Model file for the job. Use its own axes, mm. Round coordinates to 2 decimals unless told otherwise and drop trailing zeros. Order: outer loops, then holes, each group sorted by start corner. A loop starts at its lowest first (then second) coordinate and runs counter-clockwise, first axis right, second up. Notation, with made-up numbers: (62, 52.25) -> (84, 52.25) arc R19 cw to (84, 76.25) -> close; hole circle Ø5 at (-6.75, 43). An arc over 180 degrees is marked (long way). Answer as CSV lines item,"result".
Autodesk Inventor part; units mm, degrees
ref_plane "YZ Plane" through (0, 0, 0) normal (1, 0, 0) x (0, 1, 0)
ref_plane "XZ Plane" through (0, 0, 0) normal (0, 1, 0) x (-1, 0, 0)
ref_plane "XY Plane" through (0, 0, 0) normal (0, 0, 1) x (1, 0, 0)
sketch "Sketch1" plane through (0, 0, 0) normal (0, 0, 1) x (1, 0, 0)
  line L0 (-6.35, -3.6662) -> (-6.35, 3.6662)
  line L1 (-6.35, 3.6662) -> (0, 7.3323)
  line L2 (0, 7.3323) -> (6.35, 3.6662)
  line L3 (6.35, 3.6662) -> (6.35, -3.6662)
  line L4 (6.35, -3.6662) -> (0, -7.3323)
  line L5 (0, -7.3323) -> (-6.35, -3.6662)
  point P0 (0, 0)
  point P1 (0, 0)
  dimension "d0" = 12.7
extrude "Extrusion1" add sketch "Sketch1" along normal blind 73.0377
sketch "Sketch2" plane through (0, 0, 73.0377) normal (0, 0, 1) x (1, 0, 0)
  point P0 (0, 0)
  point P1 (0, 0)
hole "Hole1" at (0, 0, 73.0377) direction (0, 0, -1) diameter 3.9624 depth 13.6144 tip angle 118
sketch "Sketch3" plane through (0, 0, 0) normal (0, 0, -1) x (-1, 0, 0)
  circle A0 centre (0, 0) radius 1.9812
hole "Hole2" at (0, 0, 0) direction (0, 0, 1) diameter 3.9624 depth 13.6144 tip angle 118
properties part number "STOCK,HEX,SHAFT,TURRET,DRIVE" material "Aluminum 6061"
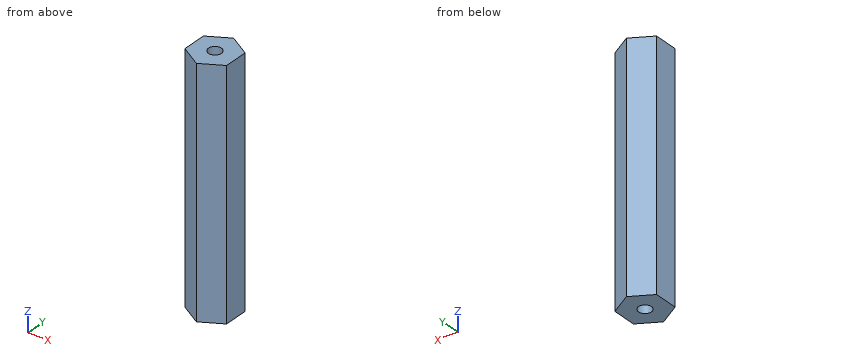
Q1. Flat gauge pins, fed straight in: pin 1 (2.5 mm diameter, centred on x = 0, y = 0, fed in from +Z); pin 2 (2 mm diameter, centred on x = -3.5, z = 46.5, fed in from +Y); pin 3 (3.5 mm diameter, centred on x = 0, y = 0, fed in from +Z). Where does each tip first touch, or does it go through?
Checks:
pin 1,"z = 58.98"
pin 2,"y = 5.89"
pin 3,"z = 59.28"
Q2. Saw through at B-B (z = 27.5). Write the cut outline in (x, y), plus the area to 3 significant figures.
Checks:
outline,"(-6.35, -3.67) -> (0, -7.33) -> (6.35, -3.67) -> (6.35, 3.67) -> (0, 7.33) -> (-6.35, 3.67) -> close"
area,"140 mm²"
Q3. Saw through at A-A (z = 60.5). Write the cut outline in (x, y).
Checks:
outline,"(-6.35, -3.67) -> (0, -7.33) -> (6.35, -3.67) -> (6.35, 3.67) -> (0, 7.33) -> (-6.35, 3.67) -> close; hole circle Ø3.96 at (0, 0)"
Q4. Wall check: L1, parallel to X at y = 0, z = 69.25; L2, parallel to Y at x = 0, z = 68.5; L3, parallel to X at y = 1.75, z = 13. Give the ranges that are in metal, low to high. Write a range as [from, to].
Checks:
L1,"[-6.35, -1.98], [1.98, 6.35]"
L2,"[-7.33, -1.98], [1.98, 7.33]"
L3,"[-6.35, -0.93], [0.93, 6.35]"
